Geometry: see drawing. Coordinates: mm, zero at the bounding-box minimum. Coordinates: 2 decimals unless noted, no trailing zeros. Write each loop counter-clockwise with the first axis right and the second up, starting at its lowest first coordinate (ties: lowest second). Pieces come first, ordered by that corner, then holes.
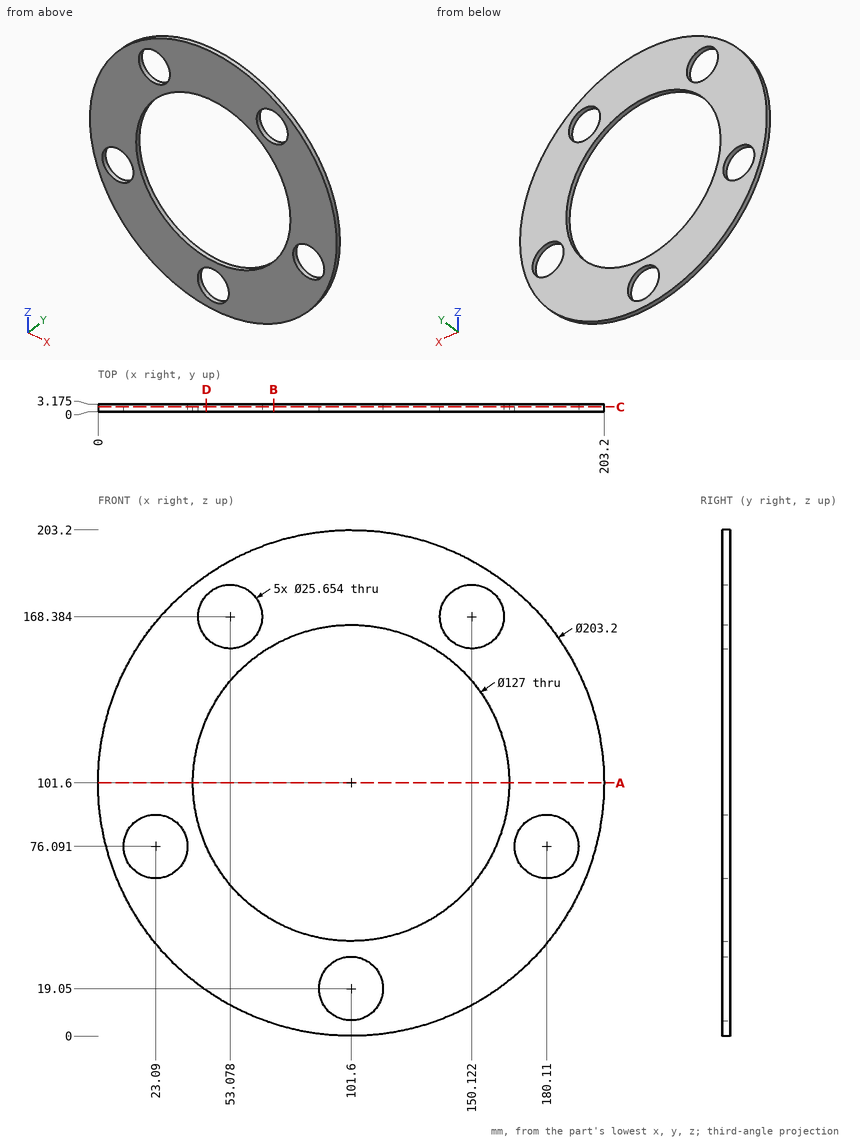
Item 1: Material intervals for probe 1 along Z at (x, y) = (101.6, 1.8); probe 2 along Z at (x, y) = (98, 2.45); probe 3 along X at (y, z) = (1.4, 81.5) (1 decimal), sorted ascending.
Derived:
probe 1: z = 0 to 6.22, 31.88 to 38.1, 165.1 to 203.2
probe 2: z = 0.06 to 6.74, 31.36 to 38.2, 165 to 203.14
probe 3: x = 2 to 11.5, 34.7 to 41.4, 161.8 to 168.5, 191.7 to 201.2
Item 2: Section A-A, the plane z = 101.6. Output: boundary loops of the cut face in (x, y) (1 decimal), plus the area to 3 significant figures.
Derived:
outline: (0, 0) - (38.1, 0) - (38.1, 3.2) - (0, 3.2) - close; (165.1, 0) - (203.2, 0) - (203.2, 3.2) - (165.1, 3.2) - close
area: 242 mm2
Item 3: Section C-C, the plane y = 2.05. State how many separate pieces and enclosed holes the cut face has, plus the area to 3 significant figures.
Derived:
separate pieces: 1
enclosed holes: 6
area: 17,200 mm2
Item 4: Pin query (flat end, axial travel): pin 1 (1.5 mm diameter, centred on y = 0.5, z = 68, fed in from +X). Return the tip coordinate at first contact, or that it passes through.
Derived:
pin 1: stops at x = 197.74
Item 5: Section B-B, the plane x = 70.5. Output: boundary loops of the cut face in (y, z) (1 decimal), plus the area to 3 significant figures.
Derived:
outline: (0, 4.9) - (3.2, 4.9) - (3.2, 46.2) - (0, 46.2) - close; (0, 157) - (3.2, 157) - (3.2, 198.3) - (0, 198.3) - close
area: 263 mm2
Item 6: Section D-D, the plane x = 43.5. Output: boundary loops of the cut face in (y, z) (1 decimal).
Derived:
outline: (0, 18.3) - (3.2, 18.3) - (3.2, 76) - (0, 76) - close; (0, 127.2) - (3.2, 127.2) - (3.2, 159.9) - (0, 159.9) - close; (0, 176.9) - (3.2, 176.9) - (3.2, 184.9) - (0, 184.9) - close
